Model file for the job. Use its own axes, mm. Coordinates: 2 decimals unless noted, no trailing zeros. Write each loop counter-clockwise with the first axis right and the second up, starting at its lowest first coordinate (ties: lowest second). Pieces come first, ordered by that corner, then holes. Notation, with made-up numbers: M -19,-31.5 L 33,-31.5 A35 ccw 33,0.5 Z; hole C 42,44.5 d9. An arc over 180 degrees is marked long. Put each result on its own line as item: value. Start each with the question number.
Q1. Drill centre lines: line 1 along X through (y, z) = (3.25, -110); line 2 along Z through (x, y) = (39, 2); line 3 along X through (y, z) = (2, -130). Where is each one in solid material? Low to high.
Q2. Cut at D-D (x = 75). Write the cut outline in (y, z), then the cut area to 3 significant figures.
Q3. Drop flat-ended pins along their axis: pin 1 (3.5 mm diameter, centred on y = 1, z = -86, fed in from +X); pin 2 (0.9 mm diameter, centred on x = 42.5, y = 8.5, fed in from -Z). Give the stop position or say it passes through.
Q4. Cut at B-B (x = 110). Write the cut outline in (y, z).
Q5. Cut at C-C (z = -70.5). Write the cut outline in (x, y), then the cut area to 3 significant figures.
Q6. Cut at A-A (z = -130). Write the cut outline in (x, y).
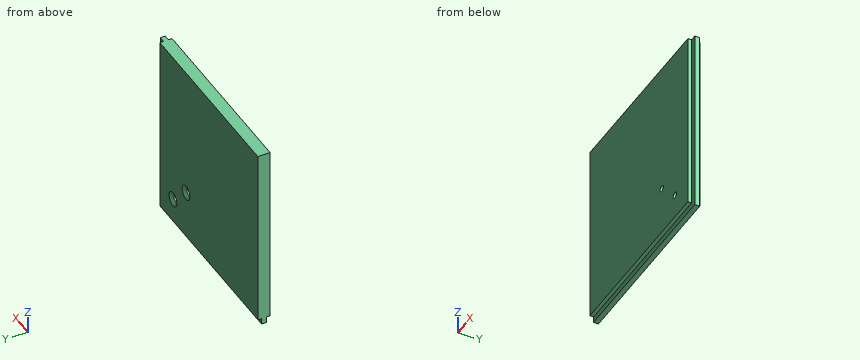
```python
from build123d import *
from OCP.BRepFilletAPI import BRepFilletAPI_MakeChamfer

# Parameters (mm, degrees)
SKETCH1_W               = 150
SKETCH1_H               = 150
BOSS_EXTRUDE1_DEPTH     = 10
SKETCH2_W               = 150
SKETCH2_H               = 4
BOSS_EXTRUDE2_DEPTH     = 5
SKETCH3_W               = 155
SKETCH3_H               = 4
BOSS_EXTRUDE3_DEPTH     = 5
CUT_EXTRUDE1_DEPTH      = 220.431082575
CUT_EXTRUDE1_DEPTH_BACK = 220.431082575
SKETCH4_R               = 2.5
CHAMFER1_SIZE           = 2
CHAMFER1_SIZE2          = 3.464101615


with BuildPart() as part:
    # Sketch1 → Boss-Extrude1 (new body)
    with BuildSketch(Plane(origin=(0, 0, 0), x_dir=(1, 0, 0), z_dir=(0, 1, 0))):
        with Locations((75, 75)):
            Rectangle(SKETCH1_W, SKETCH1_H)
    extrude(amount=BOSS_EXTRUDE1_DEPTH)

    # Sketch2 → Boss-Extrude2 (add)
    with BuildSketch(Plane(origin=(150, 0, 0), x_dir=(0, 0, -1), z_dir=(1, 0, 0))):
        with Locations((75, 5)):
            Rectangle(SKETCH2_W, SKETCH2_H)
    extrude(amount=BOSS_EXTRUDE2_DEPTH)

    # Sketch3 → Boss-Extrude3 (add)
    with BuildSketch(Plane(origin=(0, 0, -150), x_dir=(-1, 0, 0), z_dir=(0, 0, -1))):
        with Locations((-77.5, 5)):
            Rectangle(SKETCH3_W, SKETCH3_H)
    extrude(amount=BOSS_EXTRUDE3_DEPTH)

    # Sketch4 → Cut-Extrude1 (cut, two sides: drawn at the far end of the back side and taken through both)
    with BuildSketch(Plane(origin=(0, 10, 0), x_dir=(1, 0, 0), z_dir=(0, 1, 0)).offset(-CUT_EXTRUDE1_DEPTH_BACK)):
        with Locations(Location((130, 130, 0), (0, 0, 270))):
            Circle(SKETCH4_R)
        with Locations(Location((110, 110, 0), (0, 0, 270))):
            Circle(SKETCH4_R)
    extrude(amount=CUT_EXTRUDE1_DEPTH + CUT_EXTRUDE1_DEPTH_BACK, mode=Mode.SUBTRACT)

    # Chamfer1: one chamfer whose edges measure the first distance from different faces: ONE call of the kernel's chamfer builder (chamfer() names one face for all edges)
    chamfer1_edges_1 = [part.edges().sort_by_distance(p)[0] for p in [
        (130, 10, -132.5),
    ]]
    chamfer1_side_1 = [part.faces().sort_by_distance(p)[0] for p in [
        (130, 5, -132.5),
    ]]
    chamfer1_edges_2 = [part.edges().sort_by_distance(p)[0] for p in [
        (110, 10, -112.5),
    ]]
    chamfer1_side_2 = [part.faces().sort_by_distance(p)[0] for p in [
        (110, 5, -112.5),
    ]]
    chamfer1 = BRepFilletAPI_MakeChamfer(part.part.solid().wrapped)
    for e in chamfer1_edges_1:
        chamfer1.Add(CHAMFER1_SIZE, CHAMFER1_SIZE2, e.wrapped, chamfer1_side_1[0].wrapped)  # the first distance lies on this face
    for e in chamfer1_edges_2:
        chamfer1.Add(CHAMFER1_SIZE, CHAMFER1_SIZE2, e.wrapped, chamfer1_side_2[0].wrapped)  # the first distance lies on this face
    add(Compound.cast(chamfer1.Shape()), mode=Mode.REPLACE)


solid = part.part
```
Computed values:
1. line 1: 0 to 107.5, 112.5 to 155
1. line 2: -150 to 0
1. line 3: 0 to 127.5, 132.5 to 150
2. outline: M 0,-150 L 3,-150 L 3,-155 L 7,-155 L 7,-150 L 10,-150 L 10,0 L 0,0 Z
2. area: 1,520 mm2
3. pin 1: x = 150
3. pin 2: z = -150
4. outline: M 0,-150 L 3,-150 L 3,-155 L 7,-155 L 7,-150 L 10,-150 L 10,-115.96 L 8,-112.5 L 0,-112.5 Z; M 0,-107.5 L 8,-107.5 L 10,-104.04 L 10,0 L 0,0 Z
5. outline: M 0,0 L 150,0 L 150,3 L 155,3 L 155,7 L 150,7 L 150,10 L 0,10 Z
5. area: 1,520 mm2
6. outline: M 0,0 L 127.5,0 L 127.5,8 L 124.04,10 L 0,10 Z; M 132.5,0 L 150,0 L 150,3 L 155,3 L 155,7 L 150,7 L 150,10 L 135.96,10 L 132.5,8 Z
